The figure shows three views and two pictorial views of one solid part (mm, origin at its lowest corner). Answer the questions. A direction names the side the tool comes from. Round coordinates to 2 decimals unless told otherwise and drop trailing zeros. Write each loop counter-clockwise with the first axis right and the second up, starting at its lowest first coordinate (ties: lowest second). Pieces come first, ordered by that corner, then holes. Notation, with made-up numbers: (47, 49.25) - (66, 49.25) arc R32 ccw to (66, 85.25) - close; hole circle Ø6 at (73.5, 55). An arc over 180 degrees is marked (long way). Answer as CSV lines item,"result". Start each with the question number.
Item 1: Straight lines are drawn through the part: line 1 along Y through (x, z) = (20, 2.9); line 2 along Y through (x, z) = (14.5, 2.1); line 3 along X through (y, z) = (19.5, 3.75). For each, find the intervals that lie inside material, in ascending order. Write a range as [from, to].
Item 2: Which of the six approach directions +Z, -Z, +X, -X, +Y, -Y give full straight-line access (tool end or side, diameter ignored) to the marked faces 4 and 5?
Item 3: A cutting plane is placed at A-A on x = 20. Determine the outline of the cut face in (y, z).
Item 4: Flat-ended cylindrical pins translate along their axes: pin 1 (2.5 mm diameter, centred on x = 6, y = 20, fed in from +Z); pin 2 (3 mm diameter, centred on x = 9.5, z = 3.5, fed in from +Y); pin 3 (1.5 mm diameter, centred on x = 33.5, z = 3, fed in from -Y). Find the tip coordinate at first contact, or state that the pin passes through.
Item 5: A cutting plane is placed at C-C on z = 2.8. Determine the outline of the cut face in (x, y), and give its area (3 significant figures).
Item 6: A cutting plane is placed at B-B on y = 20. Determine the outline of the cut face in (x, z).
Item 7: For a pull along X with two mould halves and no side action, classify the marked faces 1, 2 and 3 as pulls with the +X half, pulls with the -X half, needs draft (parallel to the pull), parting line crosses it, or undercut.
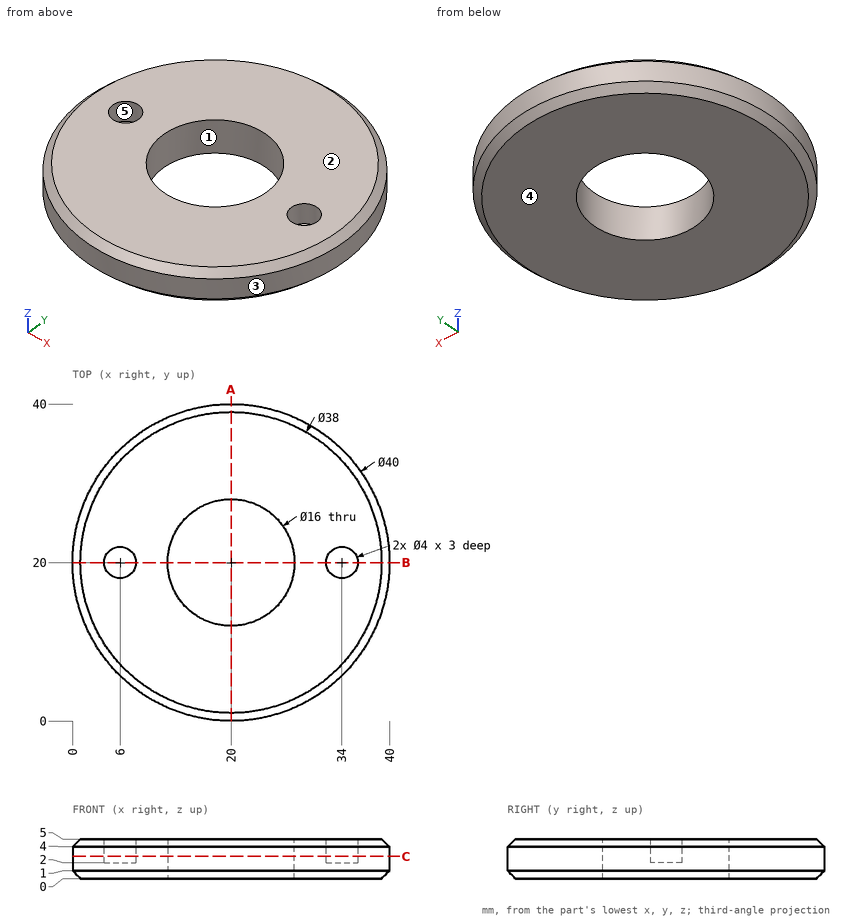
Geometry says:
1,line 1,"y = [0, 12], [28, 40]"
1,line 2,"y = [0.77, 14.19], [25.81, 39.23]"
1,line 3,"x = [0.01, 4.06], [7.94, 12.02], [27.98, 32.06], [35.94, 39.99]"
2,face 4,"-Z, +X, -X, +Y, -Y"
2,face 5,"+Z"
3,outline,"(0, 1) - (1, 0) - (12, 0) - (12, 5) - (1, 5) - (0, 4) - close; (28, 0) - (39, 0) - (40, 1) - (40, 4) - (39, 5) - (28, 5) - close"
4,pin 1,"stops at z = 2"
4,pin 2,"stops at y = 37.86"
4,pin 3,"stops at y = 4.59"
5,outline,"circle Ø40 at (20, 20); hole circle Ø4 at (6, 20); hole circle Ø16 at (20, 20); hole circle Ø4 at (34, 20)"
5,area,"1,030 mm^2"
6,outline,"(0, 1) - (1, 0) - (12, 0) - (12, 5) - (8, 5) - (8, 2) - (4, 2) - (4, 5) - (1, 5) - (0, 4) - close; (28, 0) - (39, 0) - (40, 1) - (40, 4) - (39, 5) - (36, 5) - (36, 2) - (32, 2) - (32, 5) - (28, 5) - close"
7,face 1,"undercut"
7,face 2,"needs draft"
7,face 3,"parting line crosses it"
